```python
from build123d import *

# Parameters (mm, degrees)
F0_R     = 12.7
F1_DEPTH = 38.1
F2_R     = 6.35
F3_DEPTH = 25.4
F4_R     = 6.35
F5_DEPTH = 7.62


with BuildPart() as f1:
    # F0 (on Front) → F1 (new body)
    with BuildSketch(Plane.XZ):
        with Locations((0.359142, 0)):
            Circle(F0_R)
    extrude(amount=F1_DEPTH)

    # F2 (on face) → F3 (join)
    with BuildSketch(Plane.XZ.offset(38.1)):
        Circle(F2_R)
    extrude(amount=F3_DEPTH)

    # F4 (on face) → F5 (join)
    with BuildSketch(Plane.XZ.offset(38.1)):
        Circle(F4_R)
        Polygon((-4.455793, 4.628796), (-8.695096, 3.888565), (-6.423775, 0.122331), (-8.897992, -3.39873), (-4.628796, -4.455793), (-3.888565, -8.695096), (-0.122331, -6.423775), (3.39873, -8.897992), (4.455793, -4.628796), (8.695096, -3.888565), (6.423775, -0.122331), (8.897992, 3.39873), (4.628796, 4.455793), (3.888565, 8.695096), (0.122331, 6.423775), (-3.39873, 8.897992), align=None)
        Circle(F4_R, mode=Mode.SUBTRACT)
    extrude(amount=F5_DEPTH)


solid = f1.part
```
The listing builds one solid part. Answer for the finished solid, in the listing's coordinates (mm). A direction names the side the tool comes from. Coordinates: 2 decimals unless noted, no trailing zeros. Order: outer loops, then holes, each group sorted by start corner. A loop starts at its lowest first (then second) coordinate and runs counter-clockwise, first axis right, second up. Notation, with made-up numbers: M 34,35 L 86,35 A12 cw 86,50 Z; hole C -5.5,78.25 d6. An arc over 180 degrees is marked long. Answer as a JSON object with one key per item and string values. Group by question number.
1. Section B-B on z = -5.5 is taken. Write down the section's boundary in (x, y), then the cut area to 3 significant figures.
2. Section A-A on y = -44 is taken. Write down the section's boundary in (x, z), then the cut area to 3 significant figures.
3. A tool of negligible diameter and unlimited length cuts with its end or side. For faces 1 (the flat face through (2.032, -41.857, 7.575)), 2 (the flat face through (6.546, -41.857, -4.264)), 3 (the cylindrical face through (-1.38, -54.49, -6.2)), from which of +Z, -Z, +X, -X, +Y, -Y can it reach the whole face along a straight path? Write none if from no direction.
4. Section C-C on x = -1.5 is taken. Write down the section's boundary in (y, z), then the cut area to 3 significant figures.
5. Flat-ended cylindrical pins translate along their axes: P1, Ø12, axis at y = -24.5, z = -7.5, coming from the +X side; P2, Ø12, axis at x = 1.5, y = -45.5, coming from the -Z side. Find the tip coordinate at first contact, or state that the pin passes through.
6. Section D-D on y = -33 is taken. Write down the section's boundary in (x, z), then the cut area to 3 significant figures.
7. Straight lines are drawn through the part: line 1 (Y direction, x = -7.5, z = 4.5); line 2 (Z direction, x = 0.75, y = -7); line 3 (X direction, y = -4, z = 3.5). For each, find the intervals that lie inside material, in ascending order.
8. Determine the mould class of faces 4 (the cylindrical face through (12.473, -18.783, 3.815)), 5 (the flat face through (1.61, -41.86, -7.64)), 6 (the flat face through (7.575, -41.857, -2.032)), 7 (the flat face through (-6.546, -41.857, 4.264)) for opening direction Z: released by +Z, released by -Z, zero draft, split by the parting line, or undercut.
Values follow:
{
 "1": {"outline": "M -11.09,-38.1 L -4.45,-38.1 L -4.45,-45.72 L -3.17,-45.72 L -3.17,-63.5 L 3.17,-63.5 L 3.17,-45.72 L 4.24,-45.72 L 4.24,-38.1 L 11.81,-38.1 L 11.81,0 L -11.09,0 Z", "area": "1,050 mm2"},
 "2": {"outline": "M -8.9,-3.4 L -4.63,-4.46 L -3.89,-8.7 L -0.12,-6.42 L 3.4,-8.9 L 4.46,-4.63 L 8.7,-3.89 L 6.42,-0.12 L 8.9,3.4 L 4.63,4.46 L 3.89,8.7 L 0.12,6.42 L -3.4,8.9 L -4.46,4.63 L -8.7,3.89 L -6.42,0.12 Z", "area": "187 mm2"},
 "3": {"face 1": "+Z, -Y", "face 2": "-Z, +X, -Y", "face 3": "-Y"},
 "4": {"outline": "M -63.5,-6.17 L -45.72,-6.17 L -45.72,-7.25 L -38.1,-7.25 L -38.1,-12.56 L 0,-12.56 L 0,12.56 L -38.1,12.56 L -38.1,7.56 L -45.72,7.56 L -45.72,6.17 L -63.5,6.17 Z", "area": "1,290 mm2"},
 "5": {"P1": "x = 12.97", "P2": "z = -8.9"},
 "6": {"outline": "C 0.36,0 d25.4", "area": "507 mm2"},
 "7": {"line 1": "-38.1 to 0", "line 2": "-12.69 to 12.69", "line 3": "-11.85 to 12.57"},
 "8": {"face 4": "split by the parting line", "face 5": "released by -Z", "face 6": "undercut", "face 7": "released by +Z"}
}
